```python
from build123d import *

# Parameters (mm, degrees)
SKETCH_1_W               = 90
SKETCH_1_H               = 12
EXTRUDE_1_DEPTH          = 60
CUT_EXTRUDE_1_DEPTH      = 60
SKETCH_3_R               = 9.825
EXTRUDE_2_DEPTH          = 60
CHAMFER_1_SIZE           = 2
FILLET_1_R               = 1
CHAMFER_3_SIZE           = 2
FILLET_2_R               = 5
CUT_EXTRUDE_2_REACH      = 113.467
CUT_EXTRUDE_2_END_RADIUS = 9.825
SKETCH_4_R               = 2


with BuildPart() as part:
    # Эскиз1 → Бобышка-Вытянуть1 (new body)
    with BuildSketch(Plane.XY):
        Rectangle(SKETCH_1_W, SKETCH_1_H)
    extrude(amount=EXTRUDE_1_DEPTH)

    # Эскиз2 → Вырез-Вытянуть1 (cut)
    with BuildSketch(Plane.XY.offset(60)):
        Polygon((-41, 2), (-33, -6), (27.9, -6), (35.9, 2), align=None)
    extrude(amount=-CUT_EXTRUDE_1_DEPTH, mode=Mode.SUBTRACT)

    # Эскиз3 → Бобышка-Вытянуть2 (add)
    with BuildSketch(Plane(origin=(0, 0, 0), x_dir=(-1, 0, 0), z_dir=(0, 0, -1))):
        Polygon((-73.284271247, -20), (-56.715728753, -20), (-45, -8.284271247), (-45, 8.284271247), (-56.715728753, 20), (-73.284271247, 20), (-85, 8.284271247), (-85, -8.284271247), align=None)
        with Locations((-65, 0)):
            Circle(SKETCH_3_R, mode=Mode.SUBTRACT)
    extrude(amount=-EXTRUDE_2_DEPTH)

    # Фаска1
    chamfer_1_edges = [part.edges().sort_by_distance(p)[0] for p in [
        (-45, 6, 30),
    ]]
    chamfer(chamfer_1_edges, length=CHAMFER_1_SIZE)

    # Скругление1
    fillet_1_edges = [part.edges().sort_by_distance(p)[0] for p in [
        (35.9, 2, 30),
        (-41, 2, 30),
    ]]
    fillet(fillet_1_edges, radius=FILLET_1_R)

    # Фаска3
    chamfer_3_edges = [part.edges().sort_by_distance(p)[0] for p in [
        (45, -6, 30),
        (45, 6, 30),
    ]]
    chamfer(chamfer_3_edges, length=CHAMFER_3_SIZE)

    # Скругление2
    # the kernel refuses this fillet: 5 mm, written as the material it takes off along each edge
    with BuildSketch(Plane(origin=(45, -8.284271247, -3.006121321), x_dir=(0.7071067811865452, -0.7071067811865497, 0), z_dir=(0, 0, 1))) as fillet_2_piece_1:
        with BuildLine():
            CenterArc((1.202448528, 5), FILLET_2_R, 253.698506294, 16.301493706)
            Line((-0.201010127, 0.201010127), (-0.2290793, 0.105030329))
            ThreePointArc((-0.2290793, 0.105030329), (-0.171215742, 0.029794385), (-0.070710678, -0.070710678))
            Line((-0.070710678, -0.070710678), (0, -0.1))
            Line((0, -0.1), (1.202448528, -0.1))
            Line((1.202448528, -0.1), (1.202448528, 0))
        make_face()
    extrude(amount=66.012242642, mode=Mode.SUBTRACT)
    with BuildSketch(Plane(origin=(56.715728753, -20, -5.17766953), x_dir=(1, 0, 0), z_dir=(0, 0, 1)), Plane(origin=(73.284271247, -20, -5.17766953), x_dir=(0.7071067811865485, 0.7071067811865467, 0), z_dir=(0, 0, 1)), Plane(origin=(85, -8.284271247, -5.17766953), x_dir=(0, 1, 0), z_dir=(0, 0, 1)), Plane(origin=(85, 8.284271247, -5.17766953), x_dir=(-0.7071067811865461, 0.7071067811865487, 0), z_dir=(0, 0, 1)), Plane(origin=(73.284271247, 20, -5.17766953), x_dir=(-1, 0, 0), z_dir=(0, 0, 1)), Plane(origin=(56.715728753, 20, -5.17766953), x_dir=(-0.7071067811865467, -0.7071067811865483, 0), z_dir=(0, 0, 1))) as fillet_2_piece_2:
        with BuildLine():
            CenterArc((FILLET_2_R * 0.414213562373, FILLET_2_R), FILLET_2_R, 225, 45)
            Line((-FILLET_2_R * 0.292893218813, FILLET_2_R * 0.292893218813), (-FILLET_2_R * 0.307035354437, FILLET_2_R * 0.27875108319))
            Line((-FILLET_2_R * 0.307035354437, FILLET_2_R * 0.27875108319), (-FILLET_2_R * 0.00828427124746, -FILLET_2_R * 0.02))
            Line((-FILLET_2_R * 0.00828427124746, -FILLET_2_R * 0.02), (FILLET_2_R * 0.414213562373, -FILLET_2_R * 0.02))
            Line((FILLET_2_R * 0.414213562373, -FILLET_2_R * 0.02), (FILLET_2_R * 0.414213562373, 0))
        make_face()
    extrude(amount=70.355339059, mode=Mode.SUBTRACT)
    with BuildSketch(Plane(origin=(45, 8.284271247, -3.006121321), x_dir=(0, -1, 0), z_dir=(0, 0, 1))) as fillet_2_piece_3:
        with BuildLine():
            CenterArc((2.685274397, 4.385793414), FILLET_2_R, 225, 16.301493706)
            Line((-0.850259508, 0.850259508), (-0.920970187, 0.77954883))
            Line((-0.920970187, 0.77954883), (-0.070710678, -0.070710678))
            Line((-0.070710678, -0.070710678), (0, -0.1))
            ThreePointArc((0, -0.1), (0.142135624, -0.1), (0.236251184, -0.087715868))
            Line((0.236251184, -0.087715868), (0.284271247, 0))
        make_face()
    extrude(amount=66.012242642, mode=Mode.SUBTRACT)

    # Вырез-Вытянуть2: up to this cylinder (the profile starts outside it)
    cut_extrude_2_end = Plane(origin=(65, 0, 50), z_dir=(0, 0, -1)) * Cylinder(CUT_EXTRUDE_2_END_RADIUS, 247.584, mode=Mode.PRIVATE)
    # Эскиз4 → Вырез-Вытянуть2 (cut, up to the surface)
    with BuildSketch(Plane(origin=(0, 20, 0), x_dir=(1, 0, 0), z_dir=(0, 1, 0)), mode=Mode.PRIVATE) as cut_extrude_2_sk1:
        with Locations(Location((65, -50, 0), (0, 0, 270))):
            Circle(SKETCH_4_R)
    cut_extrude_2_tool1 = extrude(cut_extrude_2_sk1.sketch, amount=-CUT_EXTRUDE_2_REACH, mode=Mode.PRIVATE) - cut_extrude_2_end
    add(cut_extrude_2_tool1.solids().sort_by_distance((65, 20, 50))[0], mode=Mode.SUBTRACT)


solid = part.part
```
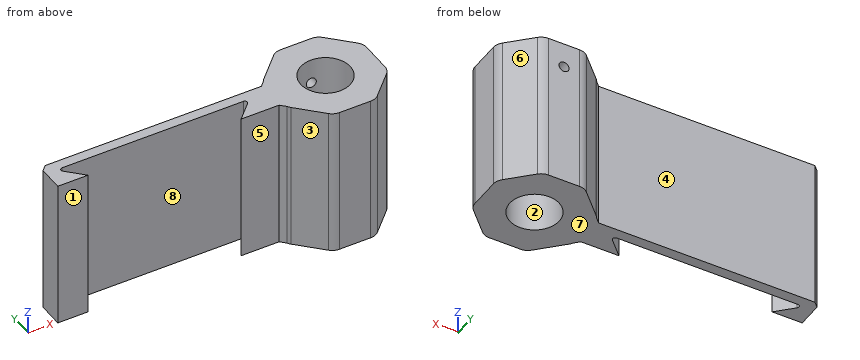
Geometry check sheet. Reference: the model listing, model coordinates, mm. Face numbers are marked on the shaded views. A direction names the side the tool comes from. Give positions to 0.01 mm unless a question says otherwise; leave off trailing zeros. Order: outer loops, then holes, each group sorted by start corner. A loop starts at its lowest first (then second) coordinate and runs counter-clockwise, first axis right, second up. Notation, with made-up numbers: (88, -32.75) - (116, -32.75) arc R17 ccw to (116, -21.75) - close; hole circle Ø7 at (51, -1.5). An arc over 180 degrees is marked (long way). Answer in a Markdown table with one row per item. Add a question column.
Q1. Cross-section at B-B, the plane z = 31.5. Enter the section's corners in (x, y) (3 decimals), then the cut area to 3 significant figures.
Q2. Material ranges on probe 1 along Y at (x, z) = (65, 44) (3 decimals); probe 2 along Z at (x, y) = (65, 17.5); probe 3 along Y at (x, z) = (18, 21), recorded low to high. Write a range as from..to.
Q3. Tool access check on the marked faces 4, 5, 6, 7 and 8. Record the directions out of +Z, -Z, +X, -X, +Y, -Y that give a thin tool (end or side, any length) a straight path to the whole face; none if there is none.
Q4. Cross-section at C-C, the plane y = -1.5. Enter the section's corners in (x, z), then the cut area to 3 significant figures.
Q5. Mould release check, pull along X, two halves, no side actions. Record for the marked faces 1, 2 and 3: pulls with the +X half, pulls with the -X half, needs draft (parallel to the pull), parting line crosses it, or undercut.
Q6. Gauge pin test, flat ends, axial feed: pin 1 (13 mm diameter, centred on x = -38.5, z = 20, fed in from -Y); pin 2 (5 mm diameter, centred on y = 14.5, z = 12, fed in from +X); pin 3 (17.5 mm diameter, centred on x = 65, y = 0, fed in from -Z); pin 4 (8 mm diameter, centred on x = 40, z = 39.5, fed in from -Y). Record the tip position at first contact, or that the pin passes through.
Q7. Cross-section at A-A, the plane x = 65. Enter the section's corners in (y, z) (3 decimals), then the cut area to 3 significant figures.
Check values:
| question | item | result |
|---|---|---|
| 1 | outline | (-45, -6) - (-33, -6) - (-39.293, 0.293) arc R1 cw to (-38.586, 2) - (33.486, 2) arc R1 cw to (34.193, 0.293) - (27.9, -6) - (43, -6) - (45, -8) arc R5 ccw to (45.85, -9.135) - (55.251, -18.536) arc R5 ccw to (58.787, -20) - (71.213, -20) arc R5 ccw to (74.749, -18.536) - (83.536, -9.749) arc R5 ccw to (85, -6.213) - (85, 6.213) arc R5 ccw to (83.536, 9.749) - (74.749, 18.536) arc R5 ccw to (71.213, 20) - (58.787, 20) arc R5 ccw to (55.251, 18.536) - (45.85, 9.135) arc R5 ccw to (45, 8) - (43, 6) - (-43, 6) - (-45, 4) - close; hole circle Ø19.65 at (65, 0) |
| 1 | area | 1,550 mm^2 |
| 2 | probe 1 | y = -20..-9.825, 9.825..20 |
| 2 | probe 2 | z = 0..48, 52..60 |
| 2 | probe 3 | y = 2..6 |
| 3 | face 4 | +Z, -Z, -X, +Y |
| 3 | face 5 | +Z, -Z, -X, -Y |
| 3 | face 6 | +Z, -Z, +X, +Y |
| 3 | face 7 | -Z, +X, -X, +Y, -Y |
| 3 | face 8 | +Z, -Z |
| 4 | outline | (-45, 0) - (-37.5, 0) - (-37.5, 60) - (-45, 60) - close; (32.4, 0) - (55.29, 0) - (55.29, 60) - (32.4, 60) - close; (74.71, 0) - (85, 0) - (85, 60) - (74.71, 60) - close |
| 4 | area | 2,440 mm^2 |
| 5 | face 1 | needs draft |
| 5 | face 2 | undercut |
| 5 | face 3 | pulls with the -X half |
| 6 | pin 1 | stops at y = -6 |
| 6 | pin 2 | stops at x = 81.28 |
| 6 | pin 3 | passes through |
| 6 | pin 4 | stops at y = -7 |
| 7 | outline | (-20, 0) - (-9.825, 0) - (-9.825, 60) - (-20, 60) - close; (9.825, 0) - (20, 0) - (20, 48) - (9.825, 48) - close; (9.825, 52) - (20, 52) - (20, 60) - (9.825, 60) - close |
| 7 | area | 1,180 mm^2 |
